```python
from build123d import *

# Parameters (mm, degrees)
SKETCH_1_R          = 1.95
EXTRUDE_1_DEPTH     = 60
SKETCH1_W           = 3
SKETCH1_H           = 3.9
BOSS_EXTRUDE1_DEPTH = 5
SKETCH2_W           = 2
SKETCH2_H           = 1.5
CUT_EXTRUDE1_DEPTH  = 3


with BuildPart() as part:
    # 草图1 → 凸台-拉伸1 (new body)
    with BuildSketch(Plane.XY):
        Circle(SKETCH_1_R)
    extrude(amount=EXTRUDE_1_DEPTH)

    # Sketch1 → Boss-Extrude1 (add)
    with BuildSketch(Plane(origin=(0, 0, 0), x_dir=(0, 0, -1), z_dir=(1, 0, 0))):
        with Locations((-32, 0)):
            Rectangle(SKETCH1_W, SKETCH1_H)
    extrude(amount=BOSS_EXTRUDE1_DEPTH)

    # Sketch2 → Cut-Extrude1 (cut)
    with BuildSketch(Plane(origin=(0, 0, 30.5), x_dir=(-1, 0, 0), z_dir=(0, 0, -1))):
        with Locations((-2.8, 1.2)):
            Rectangle(SKETCH2_W, SKETCH2_H)
    extrude(amount=-CUT_EXTRUDE1_DEPTH, mode=Mode.SUBTRACT)


solid = part.part
```
Could you check a few things on this model? Use its own coordinates, in mm. A direction names the side the tool comes from. Give positions to 0.01 mm unless a question says otherwise; leave off trailing zeros. Order: outer loops, then holes, each group sorted by start corner. A loop starts at its lowest first (then second) coordinate and runs counter-clockwise, first axis right, second up.
Q1. For faces 1 (the flat face through (3.8, 1, 32)), 2 (the flat face through (2, -1.95, 32)), 3 (the flat face through (1.4, 1.6, 30.5)), which set-ups out of +Z, -Z, +X, -X, +Y, -Y let a thin tool reach every point of the face, with its end or its side?
Q2. Suppose I cut it at A-A, the plane y = -0.75. Write out the boundary of the cut face in (x, z).
Q3. I'm going to push flat-ended pins straight in: P1, Ø0.8, axis at y = 1.5, z = 32.5, coming from the -X side; P2, Ø1, axis at x = 1, y = 1.5, coming from the -Z side; P3, Ø2, axis at x = 2, z = 38.5, coming from the +Y side; P4, Ø1, axis at y = -1.5, z = 9, coming from the +X side. Where does each tip first touch, or does it pass through?
Q4. If I drill on line 1 along Z through (x, y) = (2.25, 0.3); line 2 along X through (y, z) = (-0.05, 41); line 3 along X through (y, z) = (0.6, 32), over which ranges is the centre line in solid material (lowest first)?
Q5. Suppose I cut it at C-C, the plane x = 4.5. Write out the boundary of the cut face in (y, z), and give its area (3 significant figures).
Q6. We'd pull the mould along X, two halves only. Please class faces 4 (the flat face through (5, 0, 32)), 5 (the cylindrical face through (-1.437, 1.318, 29.58)), 6 (the flat face through (1.4, 1.6, 33.5)), 7 (the flat face through (1.8, 1, 32)): +X half, -X half, draft (parallel to the pull), parting line (faces both ways), or undercut.
Q7. Suppose I cut it at B-B, the plane z = 6. Write out the boundary of the cut face in (x, y), and give its area (3 significant figures).
Solution:
1. face 1: +Z, -Z, +Y
1. face 2: +Z, -Z, +X, -X, -Y
1. face 3: -Z, +X, +Y
2. outline: (-1.8, 0) - (1.8, 0) - (1.8, 30.5) - (5, 30.5) - (5, 33.5) - (1.8, 33.5) - (1.8, 60) - (-1.8, 60) - close
3. P1: stops at x = -1.61
3. P2: stops at z = 0
3. P3: stops at y = 1.67
3. P4: stops at x = 1.67
4. line 1: z = 30.5 to 33.5
4. line 2: x = -1.95 to 1.95
4. line 3: x = -1.86 to 1.8, 3.8 to 5
5. outline: (-1.95, 30.5) - (1.95, 30.5) - (1.95, 33.5) - (-1.95, 33.5) - close
5. area: 11.7 mm2
6. face 4: +X half
6. face 5: parting line
6. face 6: draft
6. face 7: undercut
7. outline: circle Ø3.9 at (0, 0)
7. area: 11.9 mm2
